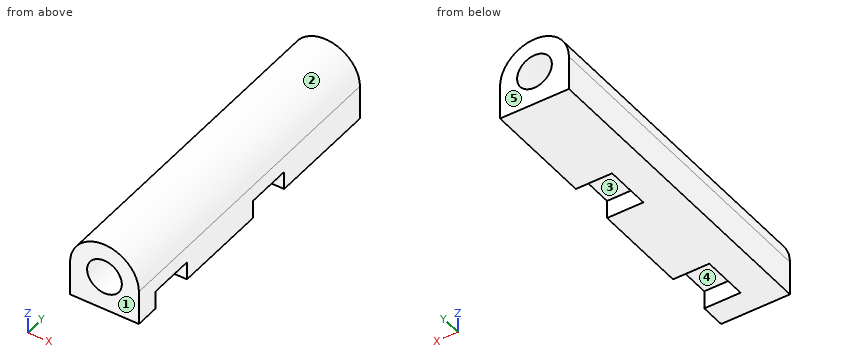
```python
from build123d import *

# Parameters (mm, degrees)
SKETCH1_R           = 3.025
BOSS_EXTRUDE1_DEPTH = 56.6
SKETCH2_W           = 8
SKETCH2_H           = 8
CUT_EXTRUDE1_DEPTH  = 3.175


with BuildPart() as part:
    # Sketch1 → Boss-Extrude1 (new body)
    with BuildSketch(Plane(origin=(0, 0, 0), x_dir=(1, 0, 0), z_dir=(0, 1, 0))):
        with BuildLine():
            Line((-6, 0), (-6, 5.43))
            Line((-6, 5.43), (-6, 6))
            Line((-6, 6), (6, 6))
            Line((6, 6), (6, 5.43))
            Line((6, 5.43), (6, 0))
            ThreePointArc((6, 0), (0, -6), (-6, 0))
        make_face()
        with Locations(Location((0, 0, 0), (0, 0, 90))):
            Circle(SKETCH1_R, mode=Mode.SUBTRACT)
    extrude(amount=BOSS_EXTRUDE1_DEPTH)

    # Sketch2 → Cut-Extrude1 (cut)
    with BuildSketch(Plane(origin=(0, 0, -6), x_dir=(-1, 0, 0), z_dir=(0, 0, -1))):
        with Locations((-3.669604029, 8.307999034)):
            Rectangle(SKETCH2_W, SKETCH2_H)
        with Locations((-3.669606205, 33.199999034)):
            Rectangle(SKETCH2_W, SKETCH2_H)
    extrude(amount=-CUT_EXTRUDE1_DEPTH, mode=Mode.SUBTRACT)


solid = part.part
```
Model file for the job. Use its own axes, mm. Face numbers are marked on the shaded views. A direction names the side the tool comes from. Round coordinates to 2 decimals unless told otherwise and drop trailing zeros. Write each loop counter-clockwise with the first axis right and the second up, starting at its lowest first coordinate (ties: lowest second). Pieces come first, ordered by that corner, then holes. Notation, with made-up numbers: (48.25, 38.5) - (72.25, 38.5) arc R37 ccw to (72.25, 74.5) - close; hole circle Ø7 at (16.5, 77.25). An arc over 180 degrees is marked (long way). One line per item, written item: value.
(1) Wall check: probe 1 along Y at (x, z) = (2, -3.5); probe 2 along X at (y, z) = (24.5, 0) (3 decimals); probe 3 along Z at (x, y) = (0, 33) (3 decimals). Give the ranges that are in metal, low to high.
Values follow:
probe 1: y = 0 to 4.31, 12.31 to 29.2, 37.2 to 56.6
probe 2: x = -6 to -3.025, 3.025 to 6
probe 3: z = 3.025 to 6
(2) Cut at C-C, the plane y = 32. Give the cut face in (x, z) (3 decimals), plus the area to 3 significant figures.
Values follow:
outline: (-6, -6) - (-0.33, -6) - (-0.33, -3.007) arc R3.025 cw (long way) to (1.082, -2.825) - (6, -2.825) - (6, 0) arc R6 ccw to (-6, 0) - close
area: 79.9 mm²
(3) 3-axis set-ups, long thin cutter, end or side, ignore diameter. For the marked faces 4 and 5: which of +Z, -Z, +X, -X, +Y, -Y reach the whole face in a straight line?
Values follow:
face 4: -Z, +X
face 5: +Z, -Z, +X, -X, +Y
(4) Cut at A-A, the plane y = 20. Give the cut face in (x, z) (3 decimals).
Values follow:
outline: (-6, -6) - (6, -6) - (6, 0) arc R6 ccw to (-6, 0) - close; hole circle Ø6.05 at (0, 0)
(5) Cut at D-D, the plane z = -0.5. Give the cut face in (x, y).
Values follow:
outline: (-6, 0) - (-2.98, 0) - (-2.98, 56.6) - (-6, 56.6) - close; (2.98, 0) - (6, 0) - (6, 56.6) - (2.98, 56.6) - close
(6) Cut at B-B, the plane x = -2. Give the cut face in (y, z), plus the area to 3 significant figures.
Values follow:
outline: (0, -6) - (56.6, -6) - (56.6, -2.27) - (0, -2.27) - close; (0, 2.27) - (56.6, 2.27) - (56.6, 5.66) - (0, 5.66) - close
area: 403 mm²
(7) Two-plate mould, pull along Y, no slides. Class the marked faces 1, 2 and 3: pulls with the +Y half, pulls with the -Y half, needs draft (parallel to the pull), parting line crosses it, or undercut.
Values follow:
face 1: pulls with the -Y half
face 2: needs draft
face 3: undercut
(8) Drop flat-ended pins along their axis: P1, Ø4, axis at y = 13, z = 4.5, coming from the +X side; P2, Ø4, axis at y = 18.5, z = 3.5, coming from the +X side; P3, Ø4, axis at x = 3.5, y = 7.5, coming from the -Z side (3 decimals); P4, Ø1, axis at x = -2, z = 1, coming from the +Y side. Give the stop position or say it passes through.
Values follow:
P1: stops at x = 5.45
P2: stops at x = 5.81
P3: stops at z = -2.825
P4: passes through
